For this review, take the finished solid that the model builds, in its own axes (mm). Face numbers are marked on the shaded views. A direction names the side the tool comes from. Give positions to 0.01 mm unless a question says otherwise; leave off trailing zeros. Loops run counter-clockwise (first coordinate to the right, second up) from the corner with the lowest first, then second, coordinate; pieces in that order, holes last.
```python
from build123d import *

# Parameters (mm, degrees)
BOSS_EXTRUDE3_DEPTH = 20
SKETCH2_W           = 10
SKETCH2_H           = 2.5
BOSS_EXTRUDE6_DEPTH = 20
SKETCH5_R           = 1.5
CUT_EXTRUDE1_DEPTH  = 20


with BuildPart() as part:
    # Sketch1 → Boss-Extrude3 (new body)
    with BuildSketch(Plane(origin=(0, 0, 0), x_dir=(1, 0, 0), z_dir=(0, 1, 0))):
        with BuildLine():
            add(Edge.make_bspline(
                [(-8.130019969, 7.5), (-11.130019969, 3.75), (-11.130019969, 0)],
                knots=[0, 0, 0, 0.5, 0.5, 0.5], degree=2))
            Line((-8.130019969, 7.5), (-13.130019969, 7.5))
            Line((-13.130019969, 7.5), (-13.130019969, -10))
            Line((-13.130019969, -10), (16.869980031, -10))
            Line((16.869980031, -10), (16.869980031, -7.5))
            Line((16.869980031, -7.5), (11.869980031, -7.5))
            Line((11.869980031, -7.5), (-8.130019969, -7.5))
            add(Edge.make_bspline(
                [(-11.130019969, 0), (-11.130019969, -3.75), (-8.130019969, -7.5)],
                knots=[0.5, 0.5, 0.5, 1, 1, 1], degree=2))
        make_face()
        with BuildLine():
            Line((-13.130019969, 7.5), (-8.130019969, 7.5))
            Line((-8.130019969, 7.5), (11.869980031, 7.5))
            add(Edge.make_bspline(
                [(11.869980031, 7.5), (14.869980031, 3.75), (14.869980031, 0)],
                knots=[0, 0, 0, 0.5, 0.5, 0.5], degree=2))
            add(Edge.make_bspline(
                [(14.869980031, 0), (14.869980031, -3.75), (11.869980031, -7.5)],
                knots=[0.5, 0.5, 0.5, 1, 1, 1], degree=2))
            Line((11.869980031, -7.5), (16.869980031, -7.5))
            Line((16.869980031, -7.5), (16.869980031, 10))
            Line((16.869980031, 10), (-13.130019969, 10))
            Line((-13.130019969, 10), (-13.130019969, 7.5))
        make_face()
    extrude(amount=BOSS_EXTRUDE3_DEPTH)

    # Sketch2 → Boss-Extrude6 (add)
    with BuildSketch(Plane(origin=(0, 20, 0), x_dir=(1, 0, 0), z_dir=(0, 1, 0))):
        with Locations((21.869980031, -8.75)):
            Rectangle(SKETCH2_W, SKETCH2_H)
        with Locations((-18.130019969, -8.75)):
            Rectangle(SKETCH2_W, SKETCH2_H)
    extrude(amount=-BOSS_EXTRUDE6_DEPTH)

    # Sketch5 → Cut-Extrude1 (cut)
    with BuildSketch(Plane(origin=(0, 0, 7.5), x_dir=(-1, 0, 0), z_dir=(0, 0, -1))):
        with Locations((18.130019969, 10)):
            Circle(SKETCH5_R)
        with Locations((-21.869980031, 10)):
            Circle(SKETCH5_R)
    extrude(amount=-CUT_EXTRUDE1_DEPTH, mode=Mode.SUBTRACT)


solid = part.part
```
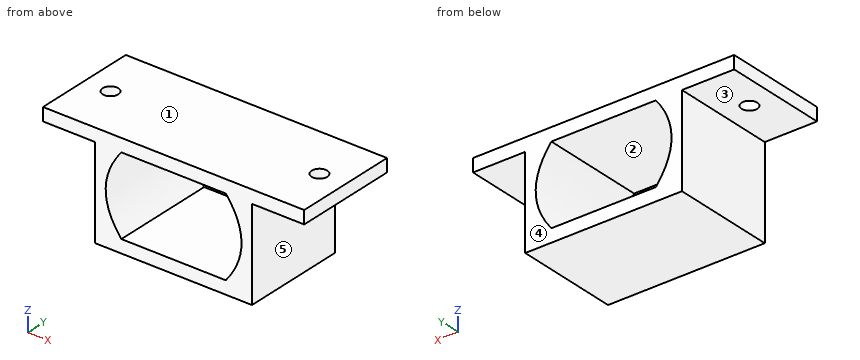
Item 1: Take a section at D-D on x = -14. Give the boundary of the cut face in (y, z).
Answer:
outline: (0, 7.5) - (20, 7.5) - (20, 10) - (0, 10) - close
Item 2: For L1, parallel to Z at x = -8, y = 4.75; L2, parallel to X at y = 5, z = 0; L3, parallel to X at y = 13, z = 6.25, list the stretches that pass through material, from the lowest coordinate up.
Answer:
L1: z = -10 to -7.5, 7.5 to 10
L2: x = -13.13 to -11.13, 14.87 to 16.87
L3: x = -13.13 to -9.05, 12.79 to 16.87
Item 3: Take a section at B-B on y = 10. State how many separate pieces and enclosed holes the cut face has, and give its area (3 significant figures).
Answer:
separate pieces: 3
enclosed holes: 1
area: 275 mm2
Item 4: Clearance check with flat-ended pins moving along their axes: pin 1 Ø5 at (x, y) = (21.87, 10) entering from -Z; pin 2 Ø1.5 at (y, z) = (10, -1.5) entering from -X. State where each tip first meets the part, or that it passes through.
Answer:
pin 1: stops at z = 7.5
pin 2: stops at x = -13.13
Item 5: Take a section at A-A on x = 7.5. Give the boundary of the cut face in (y, z).
Answer:
outline: (0, -10) - (20, -10) - (20, -7.5) - (0, -7.5) - close; (0, 7.5) - (20, 7.5) - (20, 10) - (0, 10) - close
Item 6: Take a section at C-C on x = 22. Give the boundary of the cut face in (y, z).
Answer:
outline: (0, 7.5) - (8.51, 7.5) - (8.51, 10) - (0, 10) - close; (11.49, 7.5) - (20, 7.5) - (20, 10) - (11.49, 10) - close
Item 7: Tool access review of the marked faces 1, 2, 3, 4 and 5: name each direction out of +Z, -Z, +X, -X, +Y, -Y from which nothing blocks a thin tool from reaching the whole face with its end or side.
Answer:
face 1: +Z, +X, -X, +Y, -Y
face 2: +Y, -Y
face 3: -Z, -X, +Y, -Y
face 4: +Z, -Z, +X, -X, +Y
face 5: -Z, +X, +Y, -Y
